Check sheet for the drawn part. Datum: minimum x, y, z corner. Units: mm. Coordinates: 2 decimals unless noted, no trailing zeros. Loops run counter-clockwise (first coordinate to the right, second up) from the corner with the lowest first, then second, coordinate; pieces in that order, holes last. Notation, with made-up numbers: M -14,27.25 L 16,27.25 A16 cw 16,55.25 Z; hole C -27.5,39.5 d5. An arc over 180 degrees is marked long. Use CSV: the item, a comma, the result in double quotes. Start each with the question number.
(1) Go/stop test with a flat-tipped pin: pin 1 Ø1 at (x, y) = (26, 8.5) entering from -Z. Record where the tip stops, or that it passes through.
(2) Section check A-A on x = 15. Record the cut outline in (y, z).
(3) Draft check along Z on the marked faces 1, 2, 3 and 4. Enter one of: pulls with the +Z half, pulls with the -Z half, needs draft (parallel to the pull), parting line crosses it, or undercut.
(4) Scan lines: line 1 (X direction, y = 2.25, z = 10); line 2 (Z direction, x = 13, y = 3.25); line 3 (Z direction, x = 10.5, y = 7). Record each from-to range of solid material in increasing order.
(5) Section check B-B on y = 6. Record the cut outline in (x, z).
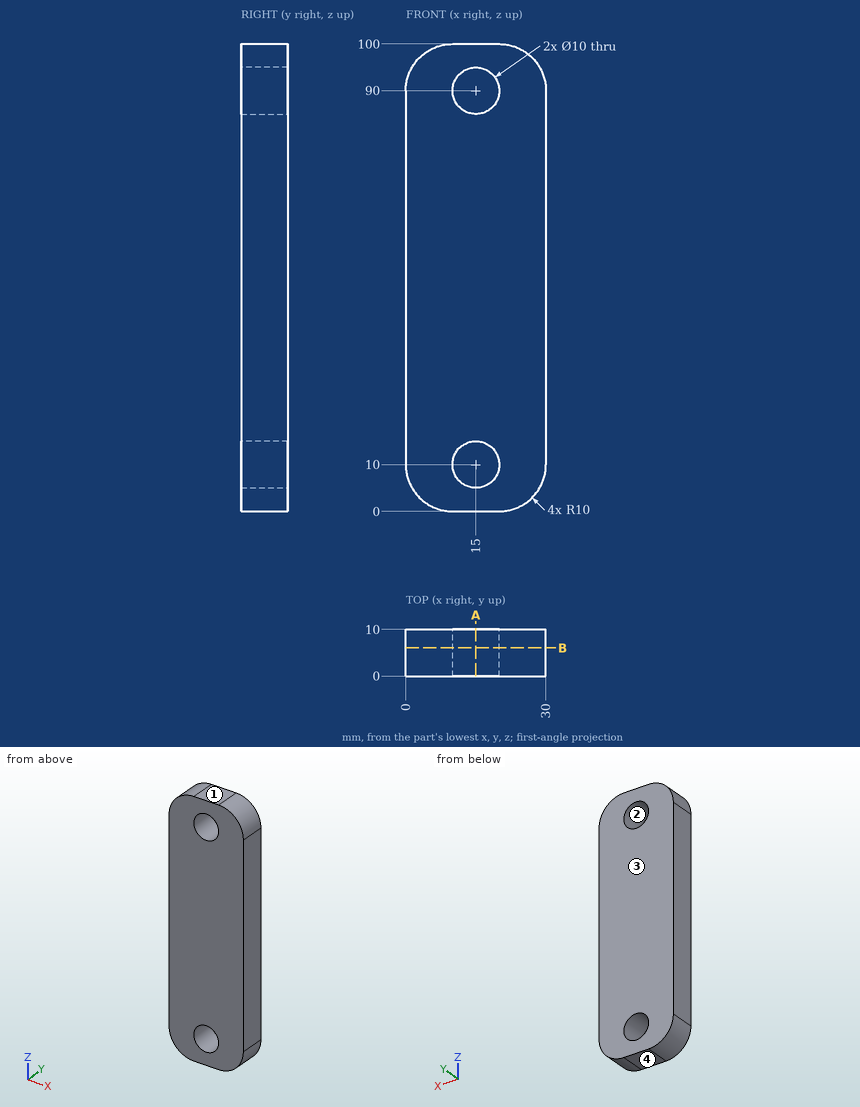
Outcome:
1,pin 1,"stops at z = 1.65"
2,outline,"M 0,0 L 10,0 L 10,5 L 0,5 Z; M 0,15 L 10,15 L 10,85 L 0,85 Z; M 0,95 L 10,95 L 10,100 L 0,100 Z"
3,face 1,"pulls with the +Z half"
3,face 2,"undercut"
3,face 3,"needs draft"
3,face 4,"pulls with the -Z half"
4,line 1,"x = 0 to 10, 20 to 30"
4,line 2,"z = 0 to 5.42, 14.58 to 85.42, 94.58 to 100"
4,line 3,"z = 0 to 7.82, 12.18 to 87.82, 92.18 to 100"
5,outline,"M 0,10 A10 ccw 10,0 L 20,0 A10 ccw 30,10 L 30,90 A10 ccw 20,100 L 10,100 A10 ccw 0,90 Z; hole C 15,10 d10; hole C 15,90 d10"
